Geometry: final body of the model. Coordinates: model frame, mm. Round coordinates to 2 decimals unless told otherwise and drop trailing zeros. Loops run counter-clockwise (first coordinate to the right, second up) from the corner with the lowest first, then second, coordinate; pieces in that order, holes last. Notation, with made-up numbers: (-28, 46.5) - (10, 46.5) arc R17 cw to (10, 79.5) - close; hole circle Ø1 at (43.25, -25.75). An arc over 180 degrees is marked (long way). Return JSON: item names as keys, results as strings. Group by question number.
1. Section A-A on z = 7. Return loops of the section in (x, y), and give its area (3 significant figures).
2. Section D-D on z = -20. Return loops of the section in (x, y), and give its area (3 significant figures).
3. Material intervals for probe 1 along Z at (x, y) = (0, 1.6); probe 2 along Z at (x, y) = (10.5, 2.2); probe 3 along X at (y, z) = (2.4, -12.8), sorted ascending.
4. Section B-B on y = 0.8. Return loops of the section in (x, z), and give its area (3 significant figures).
5. Draft query along Z for faces 1 (the face through (10.283, 1.479, -12.024)), 2 (the face through (-7.028, 1.479, -18.786)), 3 (the face through (0, 3, 2)). Return one class per face: +Z half, -Z half, draft (parallel to the pull), parting line (faces both ways), or undercut.
6. First-contact query: pin 1 Ø1.8 at (x, z) = (0, -12.8) entering from +Y; pin 2 Ø1.5 at (y, z) = (1.5, 20) entering from -X. Flat tips, straight axial feed; report the tip coordinate or a pass-through.
7. Section C-C on x = -10.5. Return loops of the section in (y, z), and give its area (3 significant figures).
from build123d import *

# Parameters (mm, degrees)
SKETCH_1_R      = 1
SKETCH_1_R_2    = 1.5
SKETCH_1_R_3    = 1.75
EXTRUDE_1_DEPTH = 3
FILLET_1_R      = 3


with BuildPart() as part:
    # 草图1 → 凸台-拉伸1 (new body)
    with BuildSketch(Plane(origin=(0, 0, 0), x_dir=(1, 0, 0), z_dir=(0, 1, 0))):
        with BuildLine():
            Line((-12.5, 15), (-12.5, -15))
            ThreePointArc((-12.5, -15), (0, -27.5), (12.5, -15))
            Line((12.5, -15), (12.5, 15))
            Line((12.5, 15), (0, 23.647980836))
            Line((0, 23.647980836), (-12.5, 15))
        make_face()
        with Locations((-10.5, 13)):
            Circle(SKETCH_1_R, mode=Mode.SUBTRACT)
        with Locations((10.5, 13)):
            Circle(SKETCH_1_R, mode=Mode.SUBTRACT)
        with Locations((0, -15)):
            Circle(SKETCH_1_R_2, mode=Mode.SUBTRACT)
        with Locations((-10.5, -7)):
            Circle(SKETCH_1_R, mode=Mode.SUBTRACT)
        with Locations((10.5, -7)):
            Circle(SKETCH_1_R, mode=Mode.SUBTRACT)
        with Locations((0, 12.8)):
            Circle(SKETCH_1_R, mode=Mode.SUBTRACT)
        with Locations((0, 20)):
            Circle(SKETCH_1_R_3, mode=Mode.SUBTRACT)
    extrude(amount=EXTRUDE_1_DEPTH)

    # 圆角1
    fillet_1_edges = [part.edges().sort_by_distance(p)[0] for p in [
        (0, 1.5, -23.647980836),
    ]]
    fillet(fillet_1_edges, radius=FILLET_1_R)


solid = part.part
Taken from the geometry:
{
 "1": {"outline": "(-12.5, 0) - (-11.5, 0) - (-11.5, 3) - (-12.5, 3) - close; (-9.5, 0) - (9.5, 0) - (9.5, 3) - (-9.5, 3) - close; (11.5, 0) - (12.5, 0) - (12.5, 3) - (11.5, 3) - close", "area": "63.0 mm2"},
 "2": {"outline": "(-5.27, 0) - (-1.75, 0) - (-1.75, 3) - (-5.27, 3) - close; (1.75, 0) - (5.27, 0) - (5.27, 3) - (1.75, 3) - close", "area": "21.1 mm2"},
 "3": {"probe 1": "-23 to -21.75, -18.25 to -13.8, -11.8 to 13.5, 16.5 to 27.5", "probe 2": "-16.38 to -14, -12 to 6, 8 to 21.78", "probe 3": "-12.5 to -11.48, -9.52 to -1, 1 to 9.52, 11.48 to 12.5"},
 "4": {"outline": "(-12.5, -15) - (-1.71, -22.47) arc R3 ccw to (1.71, -22.47) - (12.5, -15) - (12.5, 15) arc R12.5 ccw to (-12.5, 15) - close; hole circle Ø2 at (-10.5, -13); hole circle Ø2 at (-10.5, 7); hole circle Ø3.5 at (0, -20); hole circle Ø3 at (0, 15); hole circle Ø2 at (0, -12.8); hole circle Ø2 at (10.5, -13); hole circle Ø2 at (10.5, 7)", "area": "1,070 mm2"},
 "5": {"face 1": "undercut", "face 2": "-Z half", "face 3": "draft"},
 "6": {"pin 1": "through", "pin 2": "x = -11.76"},
 "7": {"outline": "(0, -16.38) - (3, -16.38) - (3, -14) - (0, -14) - close; (0, -12) - (3, -12) - (3, 6) - (0, 6) - close; (0, 8) - (3, 8) - (3, 21.78) - (0, 21.78) - close", "area": "102 mm2"}
}
